Can you work these out from the drawing? Everything is in mm from the part's minimum corner. Coordinates: 2 decimals unless noted, no trailing zeros. Write each loop counter-clockwise with the first axis right and the second up, starting at its lowest first coordinate (ties: lowest second). Pieces come first, ordered by that corner, then holes.
(1) Imagine slicing it at C-C, the plane z = 10. List the corners of the cut face in (x, y) for me, plus the area to 3 significant figures.
(2) Imagine slicing it at B-B, the plane y = 152. List the corners of the cut face in (x, z) for me, plus the area to 3 significant figures.
(3) Imagine slicing it at A-A, the plane x = 1450.5. List the corners of the cut face in (y, z) for me.
(4) For pin 1 Ø6 at (y, z) = (67.5, 6.5) entering from +X; pin 2 Ø12.5 at (y, z) = (233.5, 16.5) entering from -X, each with a flat end and sliding along its axis, tell me the tip position at first contact or that it passes through.
(5) Please list where these lines run through material, in increasing order: probe 1 along X at (y, z) = (102.5, 6.5); probe 2 along X at (y, z) = (237, 19.25); probe 3 along Y at (x, z) = (258, 1.75).
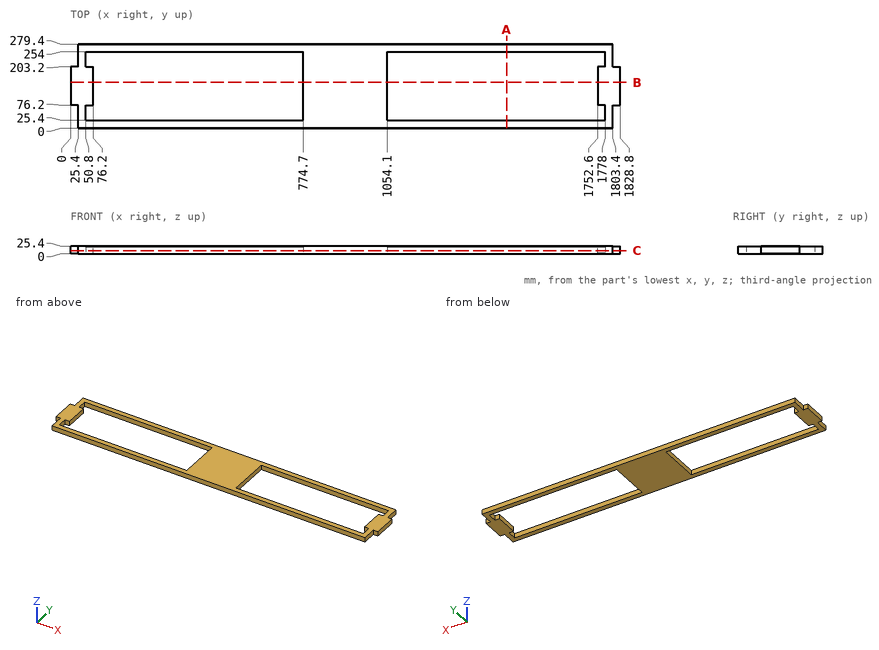
Recorded:
1. outline: (0, 76.2) - (25.4, 76.2) - (25.4, 0) - (1803.4, 0) - (1803.4, 76.2) - (1828.8, 76.2) - (1828.8, 203.2) - (1803.4, 203.2) - (1803.4, 279.4) - (25.4, 279.4) - (25.4, 203.2) - (0, 203.2) - close; hole (50.8, 25.4) - (774.7, 25.4) - (774.7, 254) - (50.8, 254) - (50.8, 203.2) - (76.2, 203.2) - (76.2, 76.2) - (50.8, 76.2) - close; hole (1054.1, 25.4) - (1778, 25.4) - (1778, 76.2) - (1752.6, 76.2) - (1752.6, 203.2) - (1778, 203.2) - (1778, 254) - (1054.1, 254) - close
1. area: 179,000 mm2
2. outline: (0, 0) - (76.2, 0) - (76.2, 25.4) - (0, 25.4) - close; (774.7, 0) - (1054.1, 0) - (1054.1, 25.4) - (774.7, 25.4) - close; (1752.6, 0) - (1828.8, 0) - (1828.8, 25.4) - (1752.6, 25.4) - close
2. area: 11,000 mm2
3. outline: (0, 0) - (25.4, 0) - (25.4, 25.4) - (0, 25.4) - close; (254, 0) - (279.4, 0) - (279.4, 25.4) - (254, 25.4) - close
4. pin 1: stops at x = 1803.4
4. pin 2: stops at x = 25.4
5. probe 1: x = 0 to 76.2, 774.7 to 1054.1, 1752.6 to 1828.8
5. probe 2: x = 25.4 to 50.8, 774.7 to 1054.1, 1778 to 1803.4
5. probe 3: y = 0 to 25.4, 254 to 279.4
